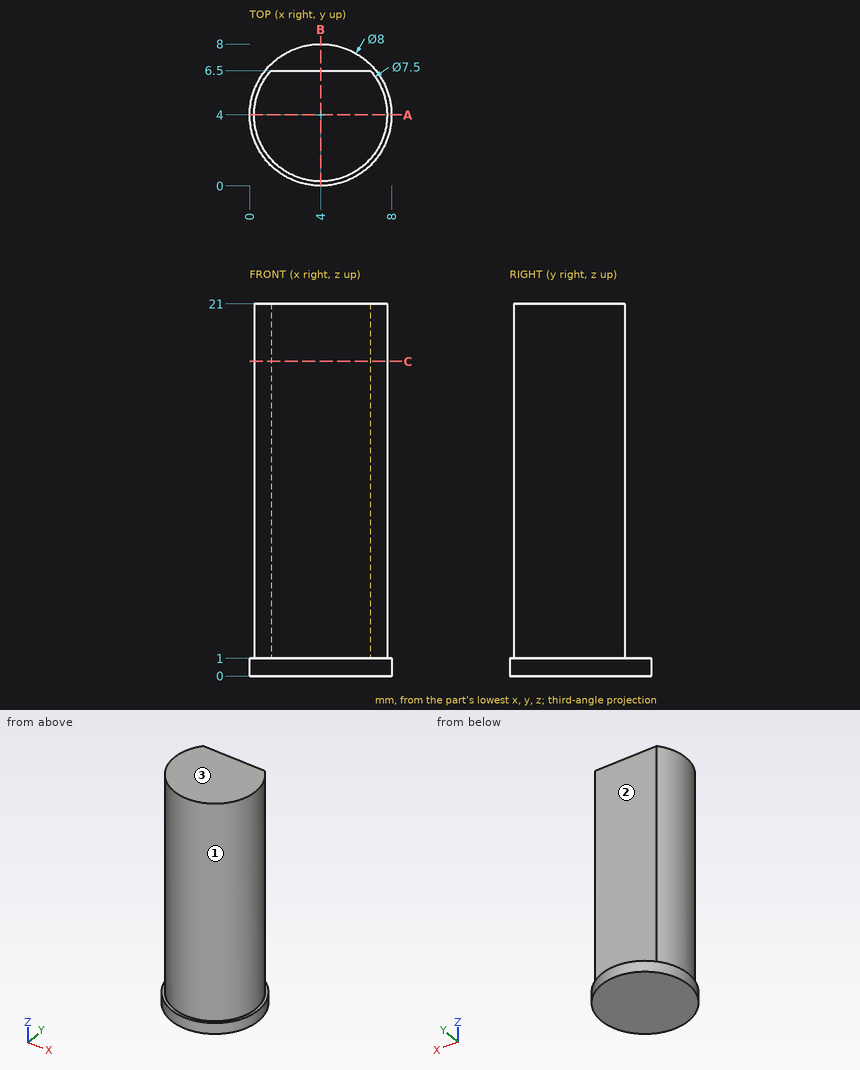
Drawing for the job (mm, zero at the part's lowest x, y, z). A direction names the side the tool comes from. Round coordinates to 2 decimals unless told otherwise and drop trailing zeros. Loops run counter-clockwise (first coordinate to the right, second up) from the corner with the lowest first, then second, coordinate; pieces in that order, holes last. Notation, with made-up numbers: (-11.75, 50.25) -> (32.25, 50.25) arc R15 cw to (32.25, 68.25) -> close; hole circle Ø2 at (54, -27). An arc over 180 degrees is marked (long way). Use one line per item in the form item = value. Start each with the question number.
Item 1: Band-saw the part on A-A (y = 4). List the corners of the cut face in (x, z), plus the area to 3 significant figures.
Item 2: Band-saw the part on B-B (x = 4). List the corners of the cut face in (y, z).
Item 3: Drop flat-ended pins along their axis: pin 1 Ø2 at (x, z) = (4.5, 13) entering from -Y; pin 2 Ø1 at (y, z) = (2.5, 16.5) entering from +X; pin 3 Ø3 at (y, z) = (6.5, 10) entering from -X. Give the stop position or say it passes through.
Item 4: Band-saw the part on C-C (z = 17.75). List the corners of the cut face in (x, y).
Item 5: Drill centre lines: line 1 along Z through (x, y) = (2, 7); line 2 along X through (y, z) = (1.5, 2.75); line 3 along Y through (x, z) = (1.5, 10.5). Where is each one in solid material? Low to high.
Item 6: Tool access for the marked faces 1, 2 and 3: list every direction of +Z, -Z, +X, -X, +Y, -Y with a clear straight run to the whole face (end or side of a thin tool).
Data:
q1.outline = (0, 0) -> (8, 0) -> (8, 1) -> (7.75, 1) -> (7.75, 21) -> (0.25, 21) -> (0.25, 1) -> (0, 1) -> close
q1.area = 158 mm^2
q2.outline = (0, 0) -> (8, 0) -> (8, 1) -> (6.5, 1) -> (6.5, 21) -> (0.25, 21) -> (0.25, 1) -> (0, 1) -> close
q3.pin_1 = 0.25
q3.pin_2 = 7.61
q3.pin_3 = 0.39
q4.outline = (1.2, 6.5) arc R3.75 ccw (long way) to (6.8, 6.5) -> close
q5.line_1 = 0 to 1
q5.line_2 = 1.2 to 6.8
q5.line_3 = 1.2 to 6.5
q6.face_1 = +Z
q6.face_2 = +Z, +X, -X, +Y
q6.face_3 = +Z, +X, -X, +Y, -Y
